```python
from build123d import *

# Parameters (mm, degrees)
SKETCH1_R           = 1.5
BOSS_EXTRUDE1_DEPTH = 3


with BuildPart() as part:
    # Sketch1 → Boss-Extrude1 (new body)
    with BuildSketch(Plane(origin=(0, 0, 0), x_dir=(0, 0, -1), z_dir=(1, 0, 0))):
        Polygon((0, -29.177050279), (-3.988546489, -29.177050279), (-3.988546489, -26.177050279), (-6.988546489, -26.177050279), (-6.988546489, -29.177050279), (-10.988546489, -29.177050279), (-10.988546489, -26.177050279), (-14.988546489, -26.177050279), (-14.988546489, -29.177050279), (-18.988546489, -29.177050279), (-18.988546489, -23.177050279), (-21.988546489, -23.177050279), (-21.988546489, -17.177050279), (-18.988546489, -17.177050279), (-18.988546489, -11.177050279), (-21.988546489, -11.177050279), (-21.988546489, -5.177050279), (-18.988546489, -5.177050279), (-18.988546489, 0.822949721), (-14.988546489, 0.822949721), (-14.988546489, -2.177050279), (-10.988546489, -2.177050279), (-10.988546489, 0.822949721), (-6.988546489, 0.822949721), (-6.988546489, -2.177050279), (-3.988546489, -2.177050279), (-3.988546489, 0.822949721), (0, 0.822949721), align=None)
        with Locations((-10, -6.917050279)):
            Circle(SKETCH1_R, mode=Mode.SUBTRACT)
        with Locations(Location((-10, -21.437050279, 0), (0, 0, 180))):
            Circle(SKETCH1_R, mode=Mode.SUBTRACT)
    extrude(amount=BOSS_EXTRUDE1_DEPTH)


solid = part.part
```
Check sheet for the modelled part. Datum: model origin and axes. Units: mm. A direction names the side the tool comes from. Round coordinates to 2 decimals unless told otherwise and drop trailing zeros. Order: outer loops, then holes, each group sorted by start corner. A loop starts at its lowest first (then second) coordinate and runs counter-clockwise, first axis right, second up.
1) Section check C-C (y = -3). Record the boundary of the cut face in (x, z), and give its area (3 significant figures).
2) Tool access check on faces 4 (the flat face through (1, -23.177, 20)), 5 (the flat face through (1, -28, 14.989)), 6 (the flat face through (1, -1, 14.989)). Record the directions out of +Z, -Z, +X, -X, +Y, -Y that give a thin tool (end or side, any length) a straight path to the whole face; none if there is none.
3) Section check D-D (z = 14.5). Record the boundary of the cut face in (x, y).
4) Section check A-A (z = 10). Record the boundary of the cut face in (x, y), and give its area (3 significant figures).
5) Go/stop test with flat-tipped pins: pin 1 Ø1.5 at (x, y) = (1.5, -1.5) entering from +Z; pin 2 Ø0.9 at (x, z) = (1.5, 21) entering from -Y; pin 3 Ø0.9 at (x, z) = (1, 5) entering from -Y. Record where each tip stops, or that it passes through.
6) Mould release check, pull along Y, two halves, no side actions. Record for faces 1 (the cylindrical face through (1.479, -22.924, 9.805)), 2 (the flat face through (1, -28, 6.989)), 3 (the flat face through (1, -5.177, 21)): +Y half, -Y half, draft (parallel to the pull), parting line (faces both ways), or undercut.
7) Scan lines: line 1 (Z direction, x = 1.15, y = -26.25); line 2 (Y direction, x = 1, z = 10); line 3 (Y direction, x = 2.7, z = 8.75). Record each from-to range of solid material in increasing order.
8) Section check B-B (x = 2.7). Give the number of separate pieces and of enclosed holes in the cut face, and give its area (3 significant figures).
Result:
1. outline: (0, 0) - (3, 0) - (3, 18.99) - (0, 18.99) - close
1. area: 57.0 mm2
2. face 4: +Z, +X, -X, -Y
2. face 5: +X, -X, -Y
2. face 6: +X, -X, +Y
3. outline: (0, -26.18) - (3, -26.18) - (3, -2.18) - (0, -2.18) - close
4. outline: (0, -29.18) - (3, -29.18) - (3, -22.94) - (0, -22.94) - close; (0, -19.94) - (3, -19.94) - (3, -8.42) - (0, -8.42) - close; (0, -5.42) - (3, -5.42) - (3, 0.82) - (0, 0.82) - close
4. area: 72.0 mm2
5. pin 1: stops at z = 18.99
5. pin 2: stops at y = -23.18
5. pin 3: stops at y = -26.18
6. face 1: undercut
6. face 2: draft
6. face 3: +Y half
7. line 1: z = 0 to 3.99, 6.99 to 10.99, 14.99 to 18.99
7. line 2: y = -29.18 to -22.94, -19.94 to -8.42, -5.42 to 0.82
7. line 3: y = -29.18 to -22.27, -20.61 to -7.75, -6.09 to 0.82
8. separate pieces: 1
8. enclosed holes: 2
8. area: 550 mm2
